For this review, use the dimensioned drawing (mm, ordinates from the lowest corner) and the shaded views. Give positions to 0.01 mm unless a question says otherwise; leave off trailing zeros. Order: outer loops, then holes, each group sorted by start corner. A loop starts at its lowest first (then second) coordinate and runs counter-clockwise, first axis right, second up. Notation, with made-up numbers: (58, 71) - (112, 71) arc R22 ccw to (112, 82) - close; hole circle Ø3 at (34, -35). An arc over 180 degrees is marked (long way). Use a Markdown table: item, result. Add a question column.
1) We need section C-C on y = 6.5. Give the number of separate pieces and of enclosed holes in the cut face, then the cut area to 3 significant figures.
2) We need section D-D on x = 141.5. Write out the cut boundary in (y, z).
3) Wall thickness on L1, parallel to Z at x = 63.5, y = 5.75; L2, parallel to Z at x = 61, y = 0.5: over which ranges is each line inside the solid? List them lowest first.
4) We need section A-A on z = 38.1. Write out the cut boundary in (x, y), then the cut area to 3 significant figures.
5) We need section B-B on x = 38.1. Write out the cut boundary in (y, z), then the cut area to 3 significant figures.
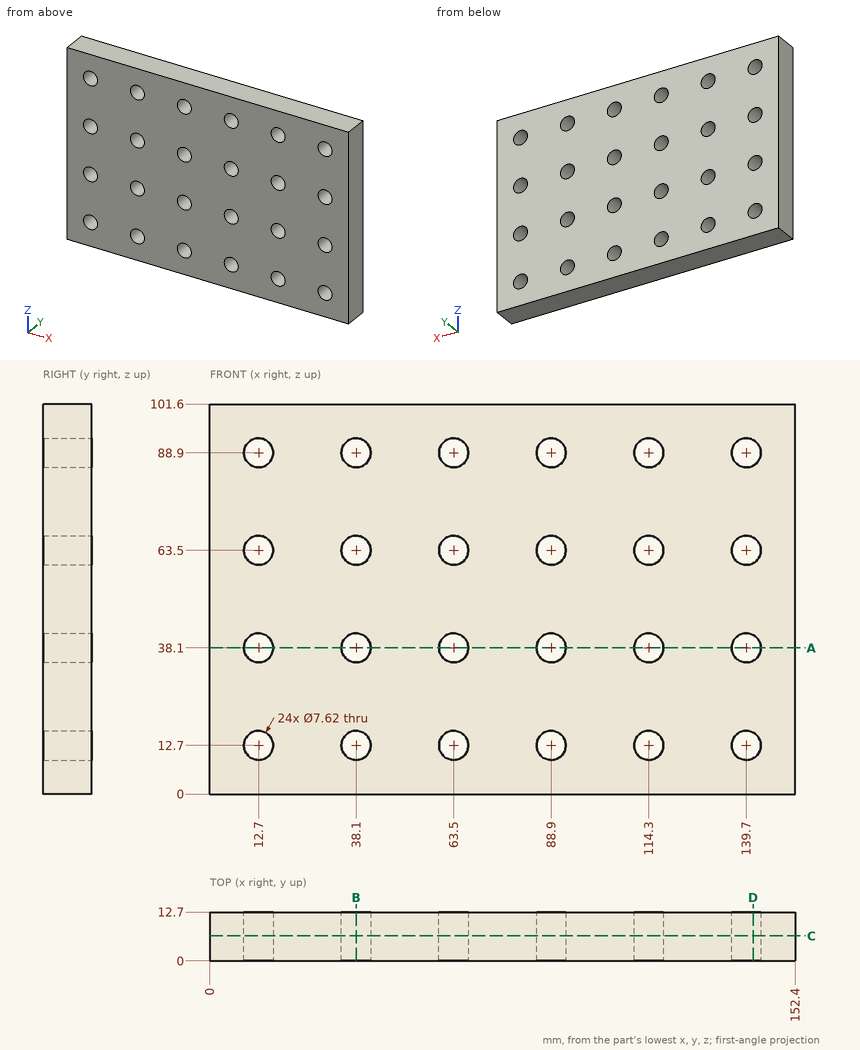
Checked values:
| question | item | result |
|---|---|---|
| 1 | separate pieces | 1 |
| 1 | enclosed holes | 24 |
| 1 | area | 14,400 mm² |
| 2 | outline | (0, 0) - (12.7, 0) - (12.7, 9.34) - (0, 9.34) - close; (0, 16.06) - (12.7, 16.06) - (12.7, 34.74) - (0, 34.74) - close; (0, 41.46) - (12.7, 41.46) - (12.7, 60.14) - (0, 60.14) - close; (0, 66.86) - (12.7, 66.86) - (12.7, 85.54) - (0, 85.54) - close; (0, 92.26) - (12.7, 92.26) - (12.7, 101.6) - (0, 101.6) - close |
| 3 | L1 | 0 to 8.89, 16.51 to 34.29, 41.91 to 59.69, 67.31 to 85.09, 92.71 to 101.6 |
| 3 | L2 | 0 to 9.82, 15.58 to 35.22, 40.98 to 60.62, 66.38 to 86.02, 91.78 to 101.6 |
| 4 | outline | (0, 0) - (8.89, 0) - (8.89, 12.7) - (0, 12.7) - close; (16.51, 0) - (34.29, 0) - (34.29, 12.7) - (16.51, 12.7) - close; (41.91, 0) - (59.69, 0) - (59.69, 12.7) - (41.91, 12.7) - close; (67.31, 0) - (85.09, 0) - (85.09, 12.7) - (67.31, 12.7) - close; (92.71, 0) - (110.49, 0) - (110.49, 12.7) - (92.71, 12.7) - close; (118.11, 0) - (135.89, 0) - (135.89, 12.7) - (118.11, 12.7) - close; (143.51, 0) - (152.4, 0) - (152.4, 12.7) - (143.51, 12.7) - close |
| 4 | area | 1,350 mm² |
| 5 | outline | (0, 0) - (12.7, 0) - (12.7, 8.89) - (0, 8.89) - close; (0, 16.51) - (12.7, 16.51) - (12.7, 34.29) - (0, 34.29) - close; (0, 41.91) - (12.7, 41.91) - (12.7, 59.69) - (0, 59.69) - close; (0, 67.31) - (12.7, 67.31) - (12.7, 85.09) - (0, 85.09) - close; (0, 92.71) - (12.7, 92.71) - (12.7, 101.6) - (0, 101.6) - close |
| 5 | area | 903 mm² |
